from build123d import *

# Parameters (mm, degrees)
SKETCH1_W           = 80
SKETCH1_H           = 50
SKETCH1_R           = 5.5
SKETCH1_R_2         = 2.5
BOSS_EXTRUDE1_DEPTH = 12.3
SKETCH2_R           = 4.6
CUT_EXTRUDE1_DEPTH  = 1.55
SKETCH3_R           = 11
CUT_EXTRUDE2_DEPTH  = 7


with BuildPart() as part:
    # Sketch1 → Boss-Extrude1 (new body)
    with BuildSketch(Plane.XY):
        with Locations((40, 25)):
            Rectangle(SKETCH1_W, SKETCH1_H)
        with Locations((40, 33.5)):
            Circle(SKETCH1_R, mode=Mode.SUBTRACT)
        with Locations((10, 30)):
            Circle(SKETCH1_R_2, mode=Mode.SUBTRACT)
        with Locations(Location((70, 30, 0), (0, 0, 180))):
            Circle(SKETCH1_R_2, mode=Mode.SUBTRACT)
        with Locations((30, 10)):
            Circle(SKETCH1_R_2, mode=Mode.SUBTRACT)
        with Locations(Location((50, 10, 0), (0, 0, 180))):
            Circle(SKETCH1_R_2, mode=Mode.SUBTRACT)
    extrude(amount=BOSS_EXTRUDE1_DEPTH)

    # Sketch2 → Cut-Extrude1 (cut)
    with BuildSketch(Plane.XY.offset(12.3)):
        with Locations((10, 30)):
            Circle(SKETCH2_R)
        with Locations((70, 30)):
            Circle(SKETCH2_R)
        with Locations((30, 10)):
            Circle(SKETCH2_R)
        with Locations((50, 10)):
            Circle(SKETCH2_R)
    extrude(amount=-CUT_EXTRUDE1_DEPTH, mode=Mode.SUBTRACT)

    # Sketch3 → Cut-Extrude2 (cut)
    with BuildSketch(Plane(origin=(0, 0, 0), x_dir=(-1, 0, 0), z_dir=(0, 0, -1))):
        with Locations((-40, 33.5)):
            Circle(SKETCH3_R)
    extrude(amount=-CUT_EXTRUDE2_DEPTH, mode=Mode.SUBTRACT)


solid = part.part
Part model, mm, in its own coordinate system. A direction names the side the tool comes from. Round coordinates to 2 decimals unless told otherwise and drop trailing zeros. Loops run counter-clockwise (first coordinate to the right, second up) from the corner with the lowest first, then second, coordinate; pieces in that order, holes last. Notation, with made-up numbers: (-20.75, 53) - (2.25, 53) arc R14 cw to (2.25, 57) - close; hole circle Ø3 at (66, 72.25). An arc over 180 degrees is marked (long way). Answer as a JSON object with one key per item and string values.
Item 1: Wall check: L1, parallel to X at y = 32, z = 6.25; L2, parallel to Y at x = 10, z = 11.75; L3, parallel to Y at x = 70, z = 4.5. Give the ranges that are in metal, low to high.
Output:
{"L1": "0 to 8.5, 11.5 to 29.1, 50.9 to 68.5, 71.5 to 80", "L2": "0 to 25.4, 34.6 to 50", "L3": "0 to 27.5, 32.5 to 50"}
Item 2: Tool access for faces 1 (the face through (54.25, 8.24, 11.54)), 2 (the face through (29.46, 7.56, 5.3)), 3 (the face through (29.839, 29.287, 3.451)): list every direction of +Z, -Z, +X, -X, +Y, -Y with a clear straight run to the whole face (end or side of a thin tool).
Output:
{"face 1": "+Z", "face 2": "+Z, -Z", "face 3": "-Z"}
Item 3: Pin check, flat tips, straight feed: pin 1 (8.5 mm diameter, centred on x = 30, y = 10, fed in from +Z); pin 2 (3 mm diameter, centred on x = 10, y = 30, fed in from -Z); pin 3 (11 mm diameter, centred on x = 40.5, y = 30, fed in from -Z). Stop position of each tip, or through.
Output:
{"pin 1": "z = 10.75", "pin 2": "through", "pin 3": "z = 7"}
Item 4: Band-saw the part on A-A on x = 70. List the corners of the cut face in (y, z), plus the area to 3 significant figures.
Output:
{"outline": "(0, 0) - (27.5, 0) - (27.5, 10.75) - (25.4, 10.75) - (25.4, 12.3) - (0, 12.3) - close; (32.5, 0) - (50, 0) - (50, 12.3) - (34.6, 12.3) - (34.6, 10.75) - (32.5, 10.75) - close", "area": "547 mm2"}
Item 5: Band-saw the part on D-D on x = 40. List the corners of the cut face in (y, z), plus the area to 3 significant figures.
Output:
{"outline": "(0, 0) - (22.5, 0) - (22.5, 7) - (28, 7) - (28, 12.3) - (0, 12.3) - close; (39, 7) - (44.5, 7) - (44.5, 0) - (50, 0) - (50, 12.3) - (39, 12.3) - close", "area": "403 mm2"}
Item 6: Band-saw the part on C-C on z = 9.25. List the corners of the cut face in (x, y), plus the area to 3 significant figures.
Output:
{"outline": "(0, 0) - (80, 0) - (80, 50) - (0, 50) - close; hole circle Ø5 at (10, 30); hole circle Ø5 at (30, 10); hole circle Ø11 at (40, 33.5); hole circle Ø5 at (50, 10); hole circle Ø5 at (70, 30)", "area": "3,830 mm2"}
Item 7: Band-saw the part on B-B on y = 30. List the corners of the cut face in (x, z), plus the area to 3 significant figures.
Output:
{"outline": "(0, 0) - (7.5, 0) - (7.5, 10.75) - (5.4, 10.75) - (5.4, 12.3) - (0, 12.3) - close; (12.5, 0) - (29.57, 0) - (29.57, 7) - (35.76, 7) - (35.76, 12.3) - (14.6, 12.3) - (14.6, 10.75) - (12.5, 10.75) - close; (44.24, 7) - (50.43, 7) - (50.43, 0) - (67.5, 0) - (67.5, 10.75) - (65.4, 10.75) - (65.4, 12.3) - (44.24, 12.3) - close; (72.5, 0) - (80, 0) - (80, 12.3) - (74.6, 12.3) - (74.6, 10.75) - (72.5, 10.75) - close", "area": "657 mm2"}
Item 8: Pull direction X, two halves, no side cores. Call faces 4 (the face through (80, 25, 6)), 5 (the face through (65.404, 30.202, 11.536)), 6 (the face through (39, 0, 6)), 7 (the face through (47.69, 10.96, 5.3)): pulls with the +X half, pulls with the -X half, needs draft (parallel to the pull), parting line crosses it, or undercut.
Output:
{"face 4": "pulls with the +X half", "face 5": "undercut", "face 6": "needs draft", "face 7": "undercut"}
